```python
from build123d import *

# Parameters (mm, degrees)
BOSS_EXTRUDE1_DEPTH = 20
DIAMETERHOLE1_D     = 9


with BuildPart() as part:
    # Sketch1 → Boss-Extrude1 (new body)
    with BuildSketch(Plane(origin=(0, 0, 0), x_dir=(0, 0, -1), z_dir=(1, 0, 0))):
        Polygon((-18, 42.5), (-18, 24), (-34.5, 24), (-35, 23.5), (-35, 0), (35, 0), (35, 23.5), (34.5, 24), (18, 24), (18, 42.5), (17.5, 43), (-17.5, 43), align=None)
    extrude(amount=BOSS_EXTRUDE1_DEPTH)

    # Sketch4 → Cut-Revolve1 (revolve, cut)
    with BuildSketch(Plane.XY, mode=Mode.PRIVATE) as cut_revolve1_sk:
        Polygon((0, 36), (6.5, 36), (6.5, 29), (13.5, 29), (13.5, 36), (20, 36), (20, 25), (0, 25), align=None)
    revolve(cut_revolve1_sk.sketch.rotate(Axis((20, 25, 0), (-1, 0, 0)), 90), axis=Axis((20, 25, 0), (-1, 0, 0)), mode=Mode.SUBTRACT)

    # DiameterHole1 (through all)
    with Locations(Plane(origin=(0, 24, 0), x_dir=(1, 0, 0), z_dir=(0, 1, 0))):
        with Locations((10, -26), (10, 26)):
            Hole(DIAMETERHOLE1_D / 2)


solid = part.part
```
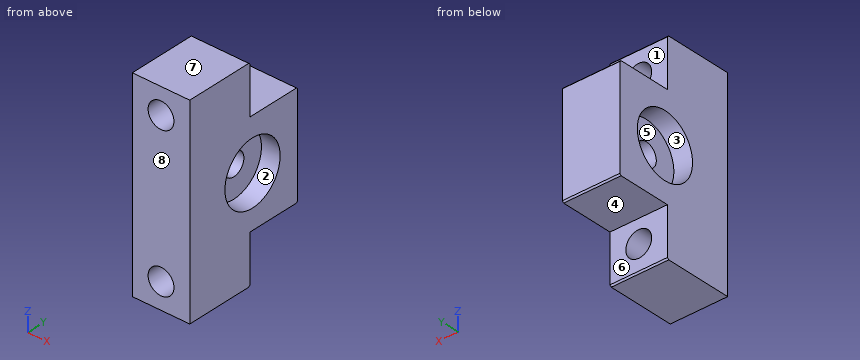
Part model, mm, in its own coordinate system. Face numbers are marked on the shaded views. A direction names the side the tool comes from. Round coordinates to 2 decimals unless told otherwise and drop trailing zeros. Loops run counter-clockwise (first coordinate to the right, second up) from the corner with the lowest first, then second, coordinate; pieces in that order, holes last.
Item 1: Mould opens along Y. For the marked faces 5, 6, 7 and 8 say: +Y half, -Y half, draft (parallel to the pull), parting line (faces both ways), or undercut.
Item 2: Cut at B-B, the plane z = 0. Give the cut face in (x, y), then the cut area to 3 significant figures.
Item 3: Cut at A-A, the plane y = 25. Give the cut face in (x, z).
Item 4: Drop flat-ended pins along their axis: P1, Ø8, axis at x = 11, z = 28.5, coming from the +Y side; P2, Ø8, axis at x = 10, z = 26, coming from the -Y side; P3, Ø13, axis at y = 25, z = 0, coming from the +X side; P4, Ø3, axis at x = 4, y = 27, coming from the -Z side. Give the stop position or say it passes through.
Item 5: Drill centre lines: line 1 (Z direction, x = 16.25, y = 25); line 2 (Z direction, x = 10, y = 16.25); line 3 (X direction, y = 5, z = -26). Where is each one in solid material? Low to high.
Item 6: 3-axis set-ups, long thin cutter, end or side, ignore diameter. For the marked faces 1, 2, 3 and 4: which of +Z, -Z, +X, -X, +Y, -Y reach the whole face in a straight line?
Item 7: Cut at D-D, the plane x = 17. Give the cut face in (y, z).
Item 8: Cut at C-C, the plane x = 10.75. Give the cut face in (y, z).
A:
1. face 5: undercut
1. face 6: +Y half
1. face 7: draft
1. face 8: -Y half
2. outline: (0, 0) - (20, 0) - (20, 14) - (13.5, 14) - (13.5, 21) - (6.5, 21) - (6.5, 14) - (0, 14) - close; (0, 36) - (6.5, 36) - (6.5, 29) - (13.5, 29) - (13.5, 36) - (20, 36) - (20, 43) - (0, 43) - close
2. area: 518 mm2
3. outline: (0, -18) - (20, -18) - (20, -11) - (13.5, -11) - (13.5, -4) - (6.5, -4) - (6.5, -11) - (0, -11) - close; (0, 11) - (6.5, 11) - (6.5, 4) - (13.5, 4) - (13.5, 11) - (20, 11) - (20, 18) - (0, 18) - close
4. P1: stops at y = 24
4. P2: passes through
4. P3: stops at x = 13.5
4. P4: stops at z = -18
5. line 1: z = -18 to -11, 11 to 18
5. line 2: z = -35 to -30.5, -21.5 to 21.5, 30.5 to 35
5. line 3: x = 0 to 5.5, 14.5 to 20
6. face 1: +Z, +X, -X, +Y
6. face 2: +X
6. face 3: -X
6. face 4: -Z, +X, -X, +Y
7. outline: (0, -35) - (23.5, -35) - (24, -34.5) - (24, -18) - (42.5, -18) - (43, -17.5) - (43, 17.5) - (42.5, 18) - (24, 18) - (24, 34.5) - (23.5, 35) - (0, 35) - close; hole circle Ø22 at (25, 0)
8. outline: (0, -35) - (23.5, -35) - (24, -34.5) - (24, -30.44) - (0, -30.44) - close; (0, -21.56) - (24, -21.56) - (24, -18) - (42.5, -18) - (43, -17.5) - (43, 17.5) - (42.5, 18) - (24, 18) - (24, 21.56) - (0, 21.56) - close; (0, 30.44) - (24, 30.44) - (24, 34.5) - (23.5, 35) - (0, 35) - close; hole circle Ø8 at (25, 0)
